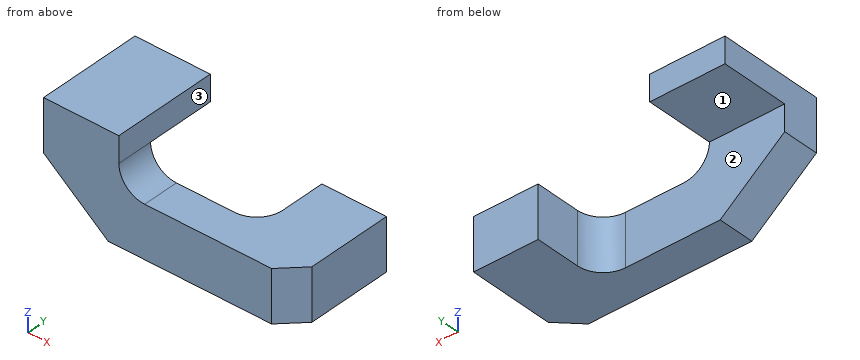
from build123d import *

# Parameters (mm, degrees)
SKETCH1_W           = 14.732
SKETCH1_H           = 6.096
BOSS_EXTRUDE1_DEPTH = 6.35
CUT_EXTRUDE2_DEPTH  = 7.35
SKETCH3_W           = 10.922
SKETCH3_H           = 6.096
CUT_EXTRUDE1_DEPTH  = 2.667
CUT_EXTRUDE3_DEPTH  = 4.683
SKETCH9_W           = 4.445
SKETCH9_H           = 1.524
BOSS_EXTRUDE2_DEPTH = 2.54
CUT_EXTRUDE4_DEPTH  = 7.096
CUT_EXTRUDE5_DEPTH  = 4.191
SKETCH15_W          = 0.048393345
SKETCH15_H          = 1.524
CUT_EXTRUDE10_DEPTH = 2.905
SKETCH13_W          = 4.445
SKETCH13_H          = 1.524
CUT_EXTRUDE11_DEPTH = 4.572


with BuildPart() as part:
    # Sketch1 → Boss-Extrude1 (new body)
    with BuildSketch(Plane(origin=(0, 0, 0), x_dir=(1, 0, 0), z_dir=(0, 1, 0))):
        Rectangle(SKETCH1_W, SKETCH1_H)
    extrude(amount=BOSS_EXTRUDE1_DEPTH)

    # Sketch4 → Cut-Extrude2 (cut, through all)
    with BuildSketch(Plane(origin=(0, 6.35, 0), x_dir=(1, 0, 0), z_dir=(0, 1, 0))):
        with BuildLine():
            Line((7.366, 0), (-1.397, 0))
            ThreePointArc((-1.397, 0), (-0.319369265, -0.446369265), (0.127, -1.524))
            ThreePointArc((0.127, -1.524), (-0.319369265, -2.601630735), (-1.397, -3.048))
            Line((-1.397, -3.048), (7.366, -3.048))
            Line((7.366, -3.048), (7.366, 0))
        make_face()
        with BuildLine():
            ThreePointArc((0.127, -1.524), (-0.319369265, -0.446369265), (-1.397, 0))
            Line((-1.397, 0), (-1.397, -3.048))
            ThreePointArc((-1.397, -3.048), (-0.319369265, -2.601630735), (0.127, -1.524))
        make_face()
        with BuildLine():
            Line((-1.397, -3.048), (-1.397, 0))
            ThreePointArc((-1.397, 0), (-2.474630735, -0.446369265), (-2.921, -1.524))
            ThreePointArc((-2.921, -1.524), (-2.474630735, -2.601630735), (-1.397, -3.048))
        make_face()
        with BuildLine():
            ThreePointArc((-1.397, -3.048), (-2.474630735, -2.601630735), (-2.921, -1.524))
            Line((-2.921, -1.524), (-2.921, -3.048))
            Line((-2.921, -3.048), (-1.397, -3.048))
        make_face()
    extrude(amount=-CUT_EXTRUDE2_DEPTH, mode=Mode.SUBTRACT)

    # Sketch3 → Cut-Extrude1 (cut)
    with BuildSketch(Plane(origin=(0, 6.35, 0), x_dir=(1, 0, 0), z_dir=(0, 1, 0))):
        with Locations((-1.905, 0)):
            Rectangle(SKETCH3_W, SKETCH3_H)
    extrude(amount=-CUT_EXTRUDE1_DEPTH, mode=Mode.SUBTRACT)

    # Sketch8 → Cut-Extrude3 (cut, through all)
    with BuildSketch(Plane(origin=(0, 3.683, 0), x_dir=(1, 0, 0), z_dir=(0, 1, 0))):
        Polygon((-7.366, 0), (-3.556, 3.048), (-7.366, 3.048), align=None)
    extrude(amount=-CUT_EXTRUDE3_DEPTH, mode=Mode.SUBTRACT)

    # Sketch9 → Boss-Extrude2 (add)
    with BuildSketch(Plane(origin=(0, 3.683, 0), x_dir=(1, 0, 0), z_dir=(0, 1, 0))):
        with Locations((-5.1435, -2.286)):
            Rectangle(SKETCH9_W, SKETCH9_H)
    extrude(amount=BOSS_EXTRUDE2_DEPTH)

    # Sketch10 → Cut-Extrude4 (cut, through all)
    with BuildSketch(Plane(origin=(0, 0, -3.048), x_dir=(-1, 0, 0), z_dir=(0, 0, -1))):
        Polygon((-7.366, 1.27), (-6.096, 0), (-7.366, 0), align=None)
    extrude(amount=-CUT_EXTRUDE4_DEPTH, mode=Mode.SUBTRACT)

    # Sketch12 → Cut-Extrude5 (cut)
    with BuildSketch(Plane(origin=(0, 0, -3.048), x_dir=(-1, 0, 0), z_dir=(0, 0, -1))):
        with BuildLine():
            ThreePointArc((-3.556, 3.683), (-3.109630735, 2.605369265), (-2.032, 2.159))
            Line((-2.032, 2.159), (2.921, 2.159))
            Line((2.921, 2.159), (2.921, 3.683))
            Line((2.921, 3.683), (-3.556, 3.683))
        make_face()
    extrude(amount=-CUT_EXTRUDE5_DEPTH, mode=Mode.SUBTRACT)

    # Sketch15 → Cut-Extrude10 (cut, through all)
    with BuildSketch(Plane(origin=(0, 0, 1.143), x_dir=(-1, 0, 0), z_dir=(0, 0, -1))):
        with Locations((2.896803328, 2.921)):
            Rectangle(SKETCH15_W, SKETCH15_H)
    extrude(amount=-CUT_EXTRUDE10_DEPTH, mode=Mode.SUBTRACT)

    # Sketch13 → Cut-Extrude11 (cut)
    with BuildSketch(Plane(origin=(0, 0, -3.048), x_dir=(-1, 0, 0), z_dir=(0, 0, -1))):
        with Locations((5.1435, 2.921)):
            Rectangle(SKETCH13_W, SKETCH13_H)
    extrude(amount=-CUT_EXTRUDE11_DEPTH, mode=Mode.SUBTRACT)


solid = part.part
The model under review builds one solid part; all positions refer to its coordinate system, in mm. Face numbers are marked on the shaded views. A direction names the side the tool comes from. Coordinates: 2 decimals unless noted, no trailing zeros. Write each loop counter-clockwise with the first axis right and the second up, starting at its lowest first coordinate (ties: lowest second). Pieces come first, ordered by that corner, then holes. Notation, with made-up numbers: (3.5, -10) - (8.5, -10) arc R21 cw to (8.5, 5) - close; hole circle Ø11 at (-25, 87). An arc over 180 degrees is marked (long way). Answer as CSV lines item,"result".
(1) For line 1 along Y through (x, z) = (0, -1.5); line 2 along X through (y, z) = (4.75, -2); line 3 along Y through (x, z) = (-4, 2), list the stretches that pass through material, from the lowest coordinate up. Write a range as [from, to].
Data:
line 1,"y = [0, 2.16]"
line 2,"x = [3.56, 7.37]"
line 3,"y = [0, 6.22]"
(2) Clearance check with flat-ended pins moving along their axes: pin 1 Ø2 at (x, z) = (-3, -0.5) entering from -Y; pin 2 Ø3.5 at (x, y) = (-5.5, 5) entering from -Z; pin 3 Ø1.2 at (x, z) = (-6, 2.5) entering from +Y; pin 4 Ø0.5 at (y, z) = (3, 2.5) entering from +X. State where each tip first meets the part, or that it passes through.
Data:
pin 1,"stops at y = 0"
pin 2,"stops at z = 1.52"
pin 3,"stops at y = 6.22"
pin 4,"stops at x = -2.92"
(3) Tool access review of the marked faces 1, 2 and 3: name each direction out of +Z, -Z, +X, -X, +Y, -Y from which nothing blocks a thin tool from reaching the whole face with its end or side.
Data:
face 1,"-Z, +X, -X, +Y"
face 2,"-Z, -X, +Y"
face 3,"+Z, +X, +Y, -Y"
(4) We need section C-C (y = 1.75). Give the boundary of the cut face in (x, z), plus the area to 3 significant figures.
Data:
outline,"(-7.37, 0) - (-3.56, -3.05) - (7.37, -3.05) - (7.37, 0) - (-1.4, 0) arc R1.52 cw to (-2.92, 1.52) - (-2.92, 3.05) - (-7.37, 3.05) - close"
area,"53.1 mm2"
(5) We need section B-B (z = -0.75). Give the boundary of the cut face in (x, y), plus the area to 3 significant figures.
Data:
outline,"(-6.43, 0) - (6.1, 0) - (7.37, 1.27) - (7.37, 6.35) - (3.56, 6.35) - (3.56, 3.68) arc R1.52 cw to (2.03, 2.16) - (-6.43, 2.16) - close"
area,"45.4 mm2"
(6) We need section A-A (y = 4.25). Give the boundary of the cut face in (x, z), plus the area to 3 significant figures.
Data:
outline,"(-7.37, 1.52) - (-2.92, 1.52) - (-2.92, 3.05) - (-7.37, 3.05) - close; (3.56, -3.05) - (7.37, -3.05) - (7.37, 0) - (3.56, 0) - close"
area,"18.4 mm2"
(7) We need section D-D (x = -1). Give the boundary of the cut face in (y, z), plus the area to 3 significant figures.
Data:
outline,"(0, -3.05) - (2.16, -3.05) - (2.16, 0) - (0, 0) - close"
area,"6.58 mm2"
